The model under review builds one solid part; all positions refer to its coordinate system, in mm. Face numbers are marked on the shaded views. A direction names the side the tool comes from. Round coordinates to 2 decimals unless told otherwise and drop trailing zeros. Order: outer loops, then holes, each group sorted by start corner. A loop starts at its lowest first (then second) coordinate and runs counter-clockwise, first axis right, second up.
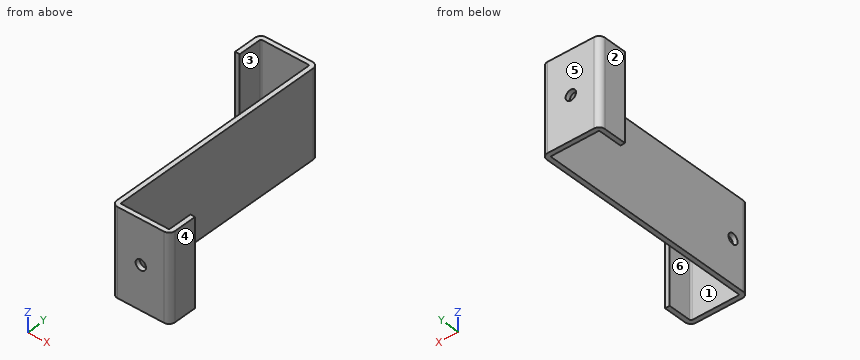
from build123d import *

# Parameters (mm, degrees)
BASEFLANGE_W                   = 75
BASEFLANGE_H                   = 200
BASE_FLANGE1_DEPTH             = 4
EDGE_FLANGE1_STRIP_W           = 18
EDGE_FLANGE1_STRIP_H           = 4
EDGE_FLANGE1_STRIP_CUT_DEPTH   = 75
EDGE_FLANGE1_STRIP_2_W         = 18
EDGE_FLANGE1_STRIP_2_H         = 4
EDGE_FLANGE1_STRIP_CUT_2_DEPTH = 75
EDGE_FLANGE1_DEPTH             = 75
EDGE_FLANGE1_BEND_DEPTH        = 75
EDGE_FLANGE2_STRIP_W           = 18
EDGE_FLANGE2_STRIP_H           = 4
EDGE_FLANGE2_STRIP_CUT_DEPTH   = 75
EDGE_FLANGE2_STRIP_2_W         = 18
EDGE_FLANGE2_STRIP_2_H         = 4
EDGE_FLANGE2_STRIP_CUT_2_DEPTH = 75
EDGE_FLANGE2_DEPTH             = 75
EDGE_FLANGE2_BEND_DEPTH        = 75
SKETCH15_R                     = 4.5
EXTRUDE1_DEPTH                 = 4
SKETCH16_R                     = 4.5
EXTRUDE2_DEPTH                 = 4
SKETCH17_R                     = 4.5
CUT_EXTRUDE1_DEPTH             = 4


# Sheet-metal steps are written as plain solids
with BuildPart() as part:
    # BaseFlange → Base-Flange1 (new body)
    with BuildSketch(Plane(origin=(0, 0, 0), x_dir=(0, 0, -1), z_dir=(1, 0, 0))):
        with Locations((0, 100)):
            Rectangle(BASEFLANGE_W, BASEFLANGE_H)
    extrude(amount=BASE_FLANGE1_DEPTH)

    # Edge-Flange1 strip (across the edge) → Edge-Flange1 strip cut (cut)
    with BuildSketch(Plane(origin=(0, 200, 37.5), x_dir=(0, -1, 0), z_dir=(0, 0, -1))):
        with Locations((-4, -2)):
            Rectangle(EDGE_FLANGE1_STRIP_W, EDGE_FLANGE1_STRIP_H)
    extrude(amount=EDGE_FLANGE1_STRIP_CUT_DEPTH, mode=Mode.SUBTRACT)

    # Edge-Flange1 strip 2 (across the edge) → Edge-Flange1 strip cut 2 (cut)
    with BuildSketch(Plane(origin=(4, 0, 37.5), x_dir=(0, 1, 0), z_dir=(0, 0, -1))):
        with Locations((-4, -2)):
            Rectangle(EDGE_FLANGE1_STRIP_2_W, EDGE_FLANGE1_STRIP_2_H)
    extrude(amount=EDGE_FLANGE1_STRIP_CUT_2_DEPTH, mode=Mode.SUBTRACT)

    # Edge-Flange1 section (across the edge) → Edge-Flange1 (add)
    with BuildSketch(Plane(origin=(0, 200, 37.5), x_dir=(0, -1, 0), z_dir=(0, 0, -1))):
        with BuildLine():
            Line((0, 1), (0, 46))
            Line((0, 46), (4, 46))
            Line((4, 46), (4, 1))
            ThreePointArc((4, 1), (4.292893219, 0.292893219), (5, 0))
            Line((5, 0), (5, -4))
            ThreePointArc((5, -4), (1.464466094, -2.535533906), (0, 1))
        make_face()
    extrude(amount=EDGE_FLANGE1_DEPTH)

    # Edge-Flange1 section 2 (across the edge) → Edge-Flange1 bend (add)
    with BuildSketch(Plane(origin=(4, 0, 37.5), x_dir=(0, 1, 0), z_dir=(0, 0, -1))):
        with BuildLine():
            Line((0, 1), (0, 46))
            Line((0, 46), (4, 46))
            Line((4, 46), (4, 1))
            ThreePointArc((4, 1), (4.292893219, 0.292893219), (5, 0))
            Line((5, 0), (5, -4))
            ThreePointArc((5, -4), (1.464466094, -2.535533906), (0, 1))
        make_face()
    extrude(amount=EDGE_FLANGE1_BEND_DEPTH)

    # Edge-Flange2 strip (across the edge) → Edge-Flange2 strip cut (cut)
    with BuildSketch(Plane(origin=(-46, 196, 37.5), x_dir=(1, 0, 0), z_dir=(0, 0, -1))):
        with Locations((-4, -2)):
            Rectangle(EDGE_FLANGE2_STRIP_W, EDGE_FLANGE2_STRIP_H)
    extrude(amount=EDGE_FLANGE2_STRIP_CUT_DEPTH, mode=Mode.SUBTRACT)

    # Edge-Flange2 strip 2 (across the edge) → Edge-Flange2 strip cut 2 (cut)
    with BuildSketch(Plane(origin=(50, 4, 37.5), x_dir=(-1, 0, 0), z_dir=(0, 0, -1))):
        with Locations((-4, -2)):
            Rectangle(EDGE_FLANGE2_STRIP_2_W, EDGE_FLANGE2_STRIP_2_H)
    extrude(amount=EDGE_FLANGE2_STRIP_CUT_2_DEPTH, mode=Mode.SUBTRACT)

    # Edge-Flange2 section (across the edge) → Edge-Flange2 (add)
    with BuildSketch(Plane(origin=(-46, 196, 37.5), x_dir=(1, 0, 0), z_dir=(0, 0, -1))):
        with BuildLine():
            Line((0, 1), (0, 21))
            Line((0, 21), (4, 21))
            Line((4, 21), (4, 1))
            ThreePointArc((4, 1), (4.292893219, 0.292893219), (5, 0))
            Line((5, 0), (5, -4))
            ThreePointArc((5, -4), (1.464466094, -2.535533906), (0, 1))
        make_face()
    extrude(amount=EDGE_FLANGE2_DEPTH)

    # Edge-Flange2 section 2 (across the edge) → Edge-Flange2 bend (add)
    with BuildSketch(Plane(origin=(50, 4, 37.5), x_dir=(-1, 0, 0), z_dir=(0, 0, -1))):
        with BuildLine():
            Line((0, 1), (0, 21))
            Line((0, 21), (4, 21))
            Line((4, 21), (4, 1))
            ThreePointArc((4, 1), (4.292893219, 0.292893219), (5, 0))
            Line((5, 0), (5, -4))
            ThreePointArc((5, -4), (1.464466094, -2.535533906), (0, 1))
        make_face()
    extrude(amount=EDGE_FLANGE2_BEND_DEPTH)

    # Sketch15 → Extrude1 (cut)
    with BuildSketch(Plane(origin=(0, 200, 0), x_dir=(1, 0, 0), z_dir=(0, 1, 0))):
        with Locations(Location((-21, 0, 0), (0, 0, 180))):
            Circle(SKETCH15_R)
    extrude(amount=-EXTRUDE1_DEPTH, mode=Mode.SUBTRACT)

    # Sketch16 → Extrude2 (cut)
    with BuildSketch(Plane.XZ):
        with Locations((25, 0)):
            Circle(SKETCH16_R)
    extrude(amount=-EXTRUDE2_DEPTH, mode=Mode.SUBTRACT)

    # Sketch17 → Cut-Extrude1 (cut)
    with BuildSketch(Plane.ZY):
        with Locations((0, 15)):
            Circle(SKETCH17_R)
    extrude(amount=-CUT_EXTRUDE1_DEPTH, mode=Mode.SUBTRACT)


solid = part.part
(1) We need section D-D (z = 24). Give the boundary of the cut face in (x, y).
(2) We need section A-A (x = 25). Give the boundary of the cut face in (y, z), and give its area (3 significant figures).
(3) Clearance check with flat-ended pins moving along their axes: P1, Ø10, axis at y = 11, z = 15.5, coming from the -X side; P2, Ø12, axis at x = 9, y = 157, coming from the +Z side; P3, Ø4.5, axis at x = 48, z = -10, coming from the +Y side; P4, Ø14.5, axis at x = 25, z = 0, coming from the +Y side. State where each tip first meets the part, or that it passes through.
(4) Tool access review of the marked faces 1, 2 and 3: name each direction out of +Z, -Z, +X, -X, +Y, -Y from which nothing blocks a thin tool from reaching the whole face with its end or side.
(5) We need section B-B (z = 0). Count the separate pieces of the cut face and the enclosed holes in it, and give its area (3 significant figures).
(6) We need section C-C (y = 15). Give the boundary of the cut face in (x, z), and give its area (3 significant figures).
(7) To check wall thickness, follow L1, parallel to Z at x = -21, y = 197; L2, parallel to X at y = 187, z = -6; L3, parallel to Y at x = -5, z = -8. State the ranges of each line that lie inside material, in increasing order.
(8) The part is to be moulded in two halves that separate along X. For the marked faces 4, 5 and 6, say which applies: pulls with the +X half, pulls with the -X half, needs draft (parallel to the pull), parting line crosses it, or undercut.
Verdict:
1. outline: (-46, 175) - (-42, 175) - (-42, 195) arc R1 cw to (-41, 196) - (-1, 196) arc R1 cw to (0, 195) - (0, 5) arc R5 ccw to (5, 0) - (45, 0) arc R5 ccw to (50, 5) - (50, 25) - (46, 25) - (46, 5) arc R1 cw to (45, 4) - (5, 4) arc R1 cw to (4, 5) - (4, 195) arc R5 ccw to (-1, 200) - (-41, 200) arc R5 ccw to (-46, 195) - close
2. outline: (0, -37.5) - (4, -37.5) - (4, -4.5) - (0, -4.5) - close; (0, 4.5) - (4, 4.5) - (4, 37.5) - (0, 37.5) - close
2. area: 264 mm2
3. P1: stops at x = 0
3. P2: stops at z = 37.5
3. P3: stops at y = 25
3. P4: stops at y = 4
4. face 1: +Z, -Z, +Y
4. face 2: +Z, -Z, -X, +Y, -Y
4. face 3: +Z, -Z, -Y
5. separate pieces: 4
5. enclosed holes: 0
5. area: 1,210 mm2
6. outline: (0, -37.5) - (4, -37.5) - (4, -4.5) - (0, -4.5) - close; (0, 4.5) - (4, 4.5) - (4, 37.5) - (0, 37.5) - close; (46, -37.5) - (50, -37.5) - (50, 37.5) - (46, 37.5) - close
6. area: 564 mm2
7. L1: z = -37.5 to -4.5, 4.5 to 37.5
7. L2: x = -46 to -42, 0 to 4
7. L3: y = 196 to 200
8. face 4: pulls with the +X half
8. face 5: needs draft
8. face 6: undercut
